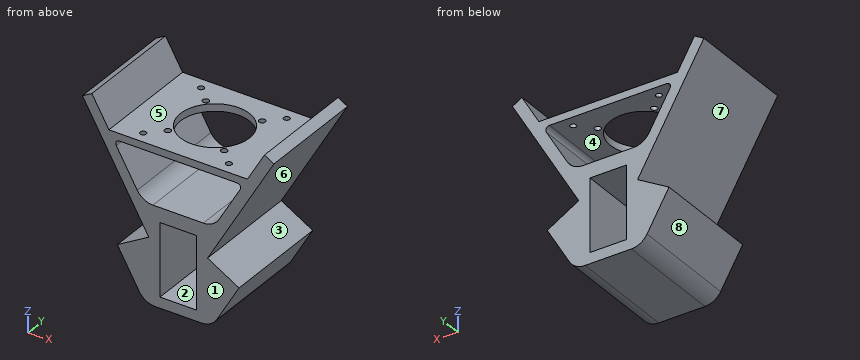
from build123d import *

# Parameters (mm, degrees)
SKETCH_1_W        = 20
SKETCH_1_H        = 40
EXTRUDE_821_DEPTH = 30
FILLET_1_R        = 10
FILLET_2_R        = 2
NEMA17_REACH      = 107.219
SKETCH_2_R        = 19
SKETCH_2_R_2      = 1.75
NEMA23_M4_REACH   = 107.219
NEMA23_M4_BORE_R  = 1.65


with BuildPart() as part:
    # Эскиз1 → Extrude 821 (new, symmetric)
    with BuildSketch(Plane(origin=(0, 0, 0), x_dir=(1, 0, 0), z_dir=(0, 1, 0))):
        Polygon((-38.118802154, -50), (38.118802154, -50), (47.483339502, -66.219854476), (52.679491924, -63.219854476), (16.179491924, 0), (33.5, 10), (18.488893001, 36), (-18.488893001, 36), (-33.5, 10), (-16.179491924, 0), (-52.679491924, -63.219854476), (-47.483339502, -66.219854476), align=None)
        Polygon((-35.809401077, -46), (-19.643593539, -18), (19.643593539, -18), (35.809401077, -46), align=None, mode=Mode.SUBTRACT)
        with Locations((0, 10)):
            Rectangle(SKETCH_1_W, SKETCH_1_H, mode=Mode.SUBTRACT)
    extrude(amount=EXTRUDE_821_DEPTH, both=True)

    # Скругление1
    fillet_1_edges = [part.edges().sort_by_distance(p)[0] for p in [
        (-18.488893001, 0, -36),
        (18.488893001, 0, -36),
        (19.643593539, 0, 18),
        (-19.643593539, 0, 18),
    ]]
    fillet(fillet_1_edges, radius=FILLET_1_R)

    # Скругление2
    fillet_2_edges = [part.edges().sort_by_distance(p)[0] for p in [
        (35.809401077, 0, 46),
        (-35.809401077, 0, 46),
    ]]
    fillet(fillet_2_edges, radius=FILLET_2_R)

    # Эскиз2 → Nema17 (cut, up to next)
    with BuildSketch(Plane.XY.offset(50), mode=Mode.PRIVATE) as nema17_sk1:
        Circle(SKETCH_2_R)
    nema17_tool1 = extrude(nema17_sk1.sketch, amount=-NEMA17_REACH, mode=Mode.PRIVATE) & part.part
    # Эскиз2 → Nema17 (cut, up to next)
    with BuildSketch(Plane.XY.offset(50), mode=Mode.PRIVATE) as nema17_sk2:
        with Locations((-15.5, 15.5)):
            Circle(SKETCH_2_R_2)
    nema17_tool2 = extrude(nema17_sk2.sketch, amount=-NEMA17_REACH, mode=Mode.PRIVATE) & part.part
    # Эскиз2 → Nema17 (cut, up to next)
    with BuildSketch(Plane.XY.offset(50), mode=Mode.PRIVATE) as nema17_sk3:
        with Locations((15.5, 15.5)):
            Circle(SKETCH_2_R_2)
    nema17_tool3 = extrude(nema17_sk3.sketch, amount=-NEMA17_REACH, mode=Mode.PRIVATE) & part.part
    # Эскиз2 → Nema17 (cut, up to next)
    with BuildSketch(Plane.XY.offset(50), mode=Mode.PRIVATE) as nema17_sk4:
        with Locations((15.5, -15.5)):
            Circle(SKETCH_2_R_2)
    nema17_tool4 = extrude(nema17_sk4.sketch, amount=-NEMA17_REACH, mode=Mode.PRIVATE) & part.part
    # Эскиз2 → Nema17 (cut, up to next)
    with BuildSketch(Plane.XY.offset(50), mode=Mode.PRIVATE) as nema17_sk5:
        with Locations((-15.5, -15.5)):
            Circle(SKETCH_2_R_2)
    nema17_tool5 = extrude(nema17_sk5.sketch, amount=-NEMA17_REACH, mode=Mode.PRIVATE) & part.part
    add(nema17_tool1.solids().sort_by_distance((0, 0, 50))[0], mode=Mode.SUBTRACT)
    add(nema17_tool2.solids().sort_by_distance((-15.5, 15.5, 50))[0], mode=Mode.SUBTRACT)
    add(nema17_tool3.solids().sort_by_distance((15.5, 15.5, 50))[0], mode=Mode.SUBTRACT)
    add(nema17_tool4.solids().sort_by_distance((15.5, -15.5, 50))[0], mode=Mode.SUBTRACT)
    add(nema17_tool5.solids().sort_by_distance((-15.5, -15.5, 50))[0], mode=Mode.SUBTRACT)

    # Nema23 - M4 bore → Nema23 - M4 (cut, up to next)
    with BuildSketch(Plane.XY.offset(50), mode=Mode.PRIVATE) as nema23_m4_sk1:
        with Locations((-23.57, 23.57)):
            Circle(NEMA23_M4_BORE_R)
    nema23_m4_tool1 = extrude(nema23_m4_sk1.sketch, amount=-NEMA23_M4_REACH, mode=Mode.PRIVATE) & part.part
    # Nema23 - M4 bore → Nema23 - M4 (cut, up to next)
    with BuildSketch(Plane.XY.offset(50), mode=Mode.PRIVATE) as nema23_m4_sk2:
        with Locations((23.57, 23.57)):
            Circle(NEMA23_M4_BORE_R)
    nema23_m4_tool2 = extrude(nema23_m4_sk2.sketch, amount=-NEMA23_M4_REACH, mode=Mode.PRIVATE) & part.part
    # Nema23 - M4 bore → Nema23 - M4 (cut, up to next)
    with BuildSketch(Plane.XY.offset(50), mode=Mode.PRIVATE) as nema23_m4_sk3:
        with Locations((23.57, -23.57)):
            Circle(NEMA23_M4_BORE_R)
    nema23_m4_tool3 = extrude(nema23_m4_sk3.sketch, amount=-NEMA23_M4_REACH, mode=Mode.PRIVATE) & part.part
    # Nema23 - M4 bore → Nema23 - M4 (cut, up to next)
    with BuildSketch(Plane.XY.offset(50), mode=Mode.PRIVATE) as nema23_m4_sk4:
        with Locations((-23.57, -23.57)):
            Circle(NEMA23_M4_BORE_R)
    nema23_m4_tool4 = extrude(nema23_m4_sk4.sketch, amount=-NEMA23_M4_REACH, mode=Mode.PRIVATE) & part.part
    add(nema23_m4_tool1.solids().sort_by_distance((-23.57, 23.57, 50))[0], mode=Mode.SUBTRACT)
    add(nema23_m4_tool2.solids().sort_by_distance((23.57, 23.57, 50))[0], mode=Mode.SUBTRACT)
    add(nema23_m4_tool3.solids().sort_by_distance((23.57, -23.57, 50))[0], mode=Mode.SUBTRACT)
    add(nema23_m4_tool4.solids().sort_by_distance((-23.57, -23.57, 50))[0], mode=Mode.SUBTRACT)


solid = part.part
Could you check a few things on this model? Use its own coordinates, in mm. Face numbers are marked on the shaded views. A direction names the side the tool comes from. Coordinates: 2 decimals unless noted, no trailing zeros. Order: outer loops, then holes, each group sorted by start corner. A loop starts at its lowest first (then second) coordinate and runs counter-clockwise, first axis right, second up. Notation, with made-up numbers: (59.5, 1) - (78.5, 1) arc R24 cw to (78.5, 38) - close; hole circle Ø2 at (35, 8). An arc over 180 degrees is marked (long way). Answer in a Markdown table with one row per item. Add a question column.
(1) On a 3-axis mill with a long thin cutter (end or side, diameter ignored), from which of +Z, -Z, +X, -X, +Y, -Y can I reach the whole of each face in a straight line? I mean the marked faces 4, 5, 6, 7 and 8. Say none if no direction works.
(2) I need wall thicknesses on L1, parallel to Y at x = -23.57, z = 48.95; L2, parallel to Y at x = 0, z = 48.2; L3, parallel to Z at x = 11, y = -22.5. Which ranges of each line are inside material? Lowest first, please.
(3) If we section it at A-A, the plane y = 23.57: State how many separate pieces and enclosed holes the cut face has, then the cut area to 3 significant figures.
(4) If we mould it in two halves opening along X, with no side actions, what happens to the marked faces 1, 2 and 3? For each: released by +X, released by -X, zero draft, split by the parting line, or undercut.
(5) If we section it at D-D, the plane z = -3.5: Please give me the cut outline in (x, y).
(6) If we section it at B-B, the plane x = -4.5: Please give me the cut outline in (y, z).
(7) Will these pins go through, and if not, where does the flat tip stop? pin 1 (4.5 mm diameter, centred on x = -23.57, y = -23.57, fed in from -Z); pin 2 (6 mm diameter, centred on x = 1, y = -8, fed in from +Z); pin 3 (8 mm diameter, centred on x = 24.5, y = -23.5, fed in from +Z).
Results are:
| question | item | result |
|---|---|---|
| 1 | face 4 | +Y, -Y |
| 1 | face 5 | +Z, +Y, -Y |
| 1 | face 6 | +X, +Y, -Y |
| 1 | face 7 | -X, +Y, -Y |
| 1 | face 8 | -Z, -X, +Y, -Y |
| 2 | L1 | y = -30 to -25.22, -21.92 to 21.92, 25.22 to 30 |
| 2 | L2 | y = -30 to -19, 19 to 30 |
| 2 | L3 | z = -36 to 18, 46 to 50 |
| 3 | separate pieces | 2 |
| 3 | enclosed holes | 1 |
| 3 | area | 2,740 mm2 |
| 4 | face 1 | zero draft |
| 4 | face 2 | undercut |
| 4 | face 3 | released by +X |
| 5 | outline | (-22.24, -30) - (-10, -30) - (-10, 30) - (-22.24, 30) - close; (10, -30) - (22.24, -30) - (22.24, 30) - (10, 30) - close |
| 6 | outline | (-30, -36) - (30, -36) - (30, -30) - (-30, -30) - close; (-30, 10) - (30, 10) - (30, 18) - (-30, 18) - close; (-30, 46) - (-18.46, 46) - (-18.46, 50) - (-30, 50) - close; (18.46, 46) - (30, 46) - (30, 50) - (18.46, 50) - close |
| 7 | pin 1 | stops at z = -31.1 |
| 7 | pin 2 | stops at z = 18 |
| 7 | pin 3 | stops at z = 50 |
